Source: CAD feature listing. Evaluate the final solid. Frame: model axes, mm. A direction names the side the tool comes from. Coordinates: 2 decimals unless noted, no trailing zeros. Order: outer loops, then holes, each group sorted by start corner. A loop starts at its lowest first (then second) coordinate and runs counter-clockwise, first axis right, second up. Notation, with made-up numbers: (63, 3.5) - (75, 3.5) arc R21 ccw to (75, 32.5) - close; hole circle Ø4 at (31.5, 69). An arc over 180 degrees is marked (long way). One line per question, with ' | ' between items. Start each with the question number.
(1) Section A-A (x = 0). Return the cut outline in (y, z), then the cut area to 3 significant figures.
(2) Draft query along X for faces 4 (the cylindrical face through (4.684, -3.792, 23.825)), 5 (the cylindrical face through (-0.138, -3.792, 27.342)), 6 (the flat face through (7.125, -1, 31)), 7 (the flat face through (0, -2.54, 28)). Return one class per face: +X half, -X half, draft (parallel to the pull), parting line (faces both ways), or undercut.
(3) Access query for faces 1 (the flat face through (-8, -1, 26.626)), 2 (the flat face through (-0.819, -1, 11)), 3 (the cylindrical face through (0.03, -1.25, 27.26)). Directions: +Z, -Z, +X, -X, +Y, -Y. A direction counts if a zero-diameter tool reaches every point of the face in a straight line with its end or side. Return the directions, or none.
(4) Section D-D (y = -4). Return the cut outline in (x, z) (3 decimals), then the cut area to 3 significant figures.
(5) Line query: line 1 along Z through (x, y) = (0, -4.3); line 2 along Z through (x, y) = (0, -1.2); line 3 along Z through (x, y) = (-7, -0.8). Output: solid intervals per line, ascending.
(6) Contact query for flat-ended pins moving along their axis: P1, Ø2, axis at y = -0.5, z = 7.5, coming from the +X side; P2, Ø2, axis at y = -2, z = 7.5, coming from the -X side; P3, Ø2, axis at x = -8, y = -1.5, coming from the -Z side; P4, Ø10.5, axis at x = 0, z = 23.2, coming from the -Y side. Output: stop coordinate, or through.
(7) Section C-C (z = 20.5). Return the cut outline in (x, y).
from build123d import *

# Parameters (mm, degrees)
F0_R     = 5.715
F0_R_2   = 4.064
F1_DEPTH = 2.54
F2_R     = 0.635
F2_R_2   = 0.4191
F3_DEPTH = 2.54
F5_DEPTH = 2.54
F7_DEPTH = 2.54
F9_DEPTH = 2.54


with BuildPart() as f1:
    # F0 (on Front) → F1 (new body)
    with BuildSketch(Plane.XZ):
        with Locations((0, 23.195567)):
            Circle(F0_R)
        with Locations((0, 23.195567)):
            Circle(F0_R_2, mode=Mode.SUBTRACT)
    extrude(amount=F1_DEPTH)

    # F2 (on face) → F3 (join)
    with BuildSketch(Plane.XZ.offset(2.54)):
        with Locations((0, 27.962195)):
            Circle(F2_R)
        with Locations((0, 27.962195)):
            Circle(F2_R_2, mode=Mode.SUBTRACT)
        with Locations((-4.766628, 23.195567)):
            Circle(F2_R)
        with Locations((-4.766628, 23.195567)):
            Circle(F2_R_2, mode=Mode.SUBTRACT)
        with Locations((0, 18.428938)):
            Circle(F2_R)
        with Locations((0, 18.428938)):
            Circle(F2_R_2, mode=Mode.SUBTRACT)
        with Locations((4.766628, 23.195567)):
            Circle(F2_R)
        with Locations((4.766628, 23.195567)):
            Circle(F2_R_2, mode=Mode.SUBTRACT)
    extrude(amount=F3_DEPTH)

    # F4 (on face) → F5 (join)
    with BuildSketch(Plane(origin=(0, 0, 0), x_dir=(-1, 0, 0), z_dir=(0, 1, 0))):
        Polygon((-7.125023, 27.259567), (0, 27.259567), (7.12503, 27.259567), (7.12503, 34.545776), (-7.125023, 34.545776), align=None)
    extrude(amount=-F5_DEPTH)

    # F6 (on face) → F7 (join)
    with BuildSketch(Plane(origin=(0, 0, 0), x_dir=(-1, 0, 0), z_dir=(0, 1, 0))):
        Polygon((0.818666, 18.264024), (0, 18.264024), (-0.818667, 18.264024), (-0.818667, 3.730329), (0.818666, 3.730329), align=None)
    extrude(amount=-F7_DEPTH)

    # F8 (on face) → F9 (join)
    with BuildSketch(Plane(origin=(0, 0, 0), x_dir=(-1, 0, 0), z_dir=(0, 1, 0))):
        with BuildLine():
            Line((-2.178273, 26.626488), (-11.233678, 26.626488))
            Line((-11.233678, 26.626488), (-11.233678, 24.87598))
            Line((-11.233678, 24.87598), (-3.700312, 24.87598))
            ThreePointArc((-3.700312, 24.87598), (-3.06684, 25.862135), (-2.178273, 26.626488))
        make_face()
        with BuildLine():
            Line((11.478047, 24.87598), (11.478047, 26.626488))
            Line((11.478047, 26.626488), (2.178273, 26.626488))
            ThreePointArc((2.178273, 26.626488), (3.06684, 25.862135), (3.700312, 24.87598))
            Line((3.700312, 24.87598), (11.478047, 24.87598))
        make_face()
    extrude(amount=-F9_DEPTH)


solid = f1.part
Response values:
1) outline: (-5.08, 17.79) - (-2.54, 17.79) - (-2.54, 3.73) - (0, 3.73) - (0, 19.13) - (-2.54, 19.13) - (-2.54, 19.06) - (-5.08, 19.06) - (-5.08, 18.85) - (-2.54, 18.85) - (-2.54, 18.01) - (-5.08, 18.01) - close; (-5.08, 27.33) - (-2.54, 27.33) - (-2.54, 27.26) - (0, 27.26) - (0, 34.55) - (-2.54, 34.55) - (-2.54, 28.6) - (-5.08, 28.6) - (-5.08, 28.38) - (-2.54, 28.38) - (-2.54, 27.54) - (-5.08, 27.54) - close | area: 59.8 mm²
2) face 4: undercut | face 5: parting line | face 6: +X half | face 7: undercut
3) face 1: -X, +Y, -Y | face 2: -Z, -X, +Y, -Y | face 3: +Y, -Y
4) outline: circle Ø1.27 at (-4.767, 23.196); circle Ø1.27 at (0, 18.429); circle Ø1.27 at (0, 27.962); circle Ø1.27 at (4.767, 23.196); hole circle Ø0.838 at (-4.767, 23.196); hole circle Ø0.838 at (0, 18.429); hole circle Ø0.838 at (0, 27.962); hole circle Ø0.838 at (4.767, 23.196) | area: 2.86 mm²
5) line 1: z = 17.79 to 18.01, 18.85 to 19.06, 27.33 to 27.54, 28.38 to 28.6 | line 2: z = 3.73 to 19.13, 27.26 to 34.55 | line 3: z = 24.88 to 26.63, 27.26 to 34.55
6) P1: stops at x = 0.82 | P2: stops at x = -0.82 | P3: stops at z = 24.88 | P4: stops at y = -5.08
7) outline: (-5.04, -2.54) - (-3.04, -2.54) - (-3.04, 0) - (-5.04, 0) - close; (3.04, -2.54) - (5.04, -2.54) - (5.04, 0) - (3.04, 0) - close
